```python
from build123d import *

# Parameters (mm, degrees)
ESQUISSE1_R        = 1.1
ESQUISSE1_W        = 6.844485425
ESQUISSE1_H        = 3
BOSS_EXTRU_1_DEPTH = 0.4
ESQUISSE3_W        = 10.5
ESQUISSE3_H        = 4.6
BOSS_EXTRU_3_DEPTH = 5.8
ESQUISSE4_W        = 3.029083023
ESQUISSE4_H        = 3
BOSS_EXTRU_4_DEPTH = 5
CONG_1_R           = 0.25


with BuildPart() as part:
    # Esquisse1 → Boss.-Extru.1 (new body)
    with BuildSketch(Plane.XY):
        with BuildLine():
            Line((-5.25, -2.9), (5.25, -2.9))
            Line((5.25, -2.9), (5.25, -2.4))
            Line((5.25, -2.4), (9.35, -2.4))
            ThreePointArc((9.35, -2.4), (9.703553391, -2.253553391), (9.85, -1.9))
            Line((9.85, -1.9), (9.85, 1.9))
            ThreePointArc((9.85, 1.9), (9.703553391, 2.253553391), (9.35, 2.4))
            Line((9.35, 2.4), (5.25, 2.4))
            Line((5.25, 2.4), (5.25, 2.9))
            Line((5.25, 2.9), (-5.25, 2.9))
            Line((-5.25, 2.9), (-5.25, 2.4))
            Line((-5.25, 2.4), (-9.35, 2.4))
            ThreePointArc((-9.35, 2.4), (-9.703553391, 2.253553391), (-9.85, 1.9))
            Line((-9.85, 1.9), (-9.85, -1.9))
            ThreePointArc((-9.85, -1.9), (-9.703553391, -2.253553391), (-9.35, -2.4))
            Line((-9.35, -2.4), (-5.25, -2.4))
            Line((-5.25, -2.4), (-5.25, -2.9))
        make_face()
        with Locations((-7.001967481, 0)):
            Circle(ESQUISSE1_R, mode=Mode.SUBTRACT)
        with Locations((6.936303644, 0)):
            Circle(ESQUISSE1_R, mode=Mode.SUBTRACT)
        with Locations((-0.061879176, 0)):
            Rectangle(ESQUISSE1_W, ESQUISSE1_H, mode=Mode.SUBTRACT)
    extrude(amount=BOSS_EXTRU_1_DEPTH)

    # Esquisse3 → Boss.-Extru.3 (add)
    with BuildSketch(Plane(origin=(0, 2.9, 0), x_dir=(1, 0, 0), z_dir=(0, 1, 0))):
        with Locations((0, -2.7)):
            Rectangle(ESQUISSE3_W, ESQUISSE3_H)
    extrude(amount=-BOSS_EXTRU_3_DEPTH)

    # Esquisse4 → Boss.-Extru.4 (add)
    with BuildSketch(Plane(origin=(0, 0, 0.4), x_dir=(-1, 0, 0), z_dir=(0, 0, -1))):
        with Locations((1.514541512, 0)):
            Rectangle(ESQUISSE4_W, ESQUISSE4_H)
    extrude(amount=BOSS_EXTRU_4_DEPTH)

    # Congé1
    cong_1_edges = [part.edges().sort_by_distance(p)[0] for p in [
        (-3.029083023, 0, -4.6),
        (0, 0, -4.6),
    ]]
    fillet(cong_1_edges, radius=CONG_1_R)


solid = part.part
```
Geometry: final body of the model. Coordinates: model frame, mm. A direction names the side the tool comes from. Round coordinates to 2 decimals unless told otherwise and drop trailing zeros. Write each loop counter-clockwise with the first axis right and the second up, starting at its lowest first coordinate (ties: lowest second). Pieces come first, ordered by that corner, then holes. Notation, with made-up numbers: M -16.5,50 L 7.5,50 A7 ccw 7.5,63 Z; hole C 80.5,51.5 d2. An arc over 180 degrees is marked long. Answer in a Markdown table with one row per item. Add a question column.
(1) Contact query for flat-ended pins moving along their axis: pin 1 (1.4 mm diameter, centred on x = -7.5, y = 0.5, fed in from +Z); pin 2 (2.5 mm diameter, centred on x = -1, z = -2, fed in from +Y); pin 3 (3.5 mm diameter, centred on x = -1, z = -2.5, fed in from -Y); pin 4 (1.8 mm diameter, centred on x = -7, y = 0, fed in from -Z). Output: stop coordinate, or through.
(2) Cut plane D-D, the plane z = 3.75. Return the cut outline in (x, y).
(3) Cut plane C-C, the plane y = -0.9. Return the cut outline in (x, z).
(4) Cut plane A-A, the plane y = 0. Return the cut outline in (x, z), then the cut area to 3 significant figures.
(5) Ray query, L1, parallel to Z at x = -3.25, y = -1; L2, parallel to Z at x = 6, y = -1.9; L3, parallel to X at y = -1.1, z = 1.5. Return the intervals inside material, ascending.
(6) Draft query along Y for faces 6 (the face through (-1, -1.5, -2)), 7 (the face through (-8.1, 0, 0.2)), 8 (the face through (7.986, 0.33, 0.197)), 9 (the face through (8, 1, 0.4)). Return one class per face: pulls with the +Y half, pulls with the -Y half, needs draft (parallel to the pull), parting line crosses it, or undercut.
(7) Cut plane B-B, the plane x = -1.5. Return the cut outline in (y, z), then the cut area to 3 significant figures.
(8) Reachability of faces 1 (the face through (0, 0, 5)), 2 (the face through (2, 0, 0.4)), 3 (the face through (-1, 1.5, -2)), 4 (the face through (-8, 1, 0.4)), 5 (the face through (0, -2.9, 2)) from +Z, -Z, +X, -X, +Y, -Y: full face, straight path, thin tool, end or side. Return the list, or none.
Established:
| question | item | result |
|---|---|---|
| 1 | pin 1 | z = 0.4 |
| 1 | pin 2 | y = 1.5 |
| 1 | pin 3 | y = -1.5 |
| 1 | pin 4 | through |
| 2 | outline | M -5.25,-2.9 L 5.25,-2.9 L 5.25,2.9 L -5.25,2.9 Z |
| 3 | outline | M -9.85,0 L -7.63,0 L -7.63,0.4 L -9.85,0.4 Z; M -6.37,0 L -3.48,0 L -3.48,0.4 L -3.03,0.4 L -3.03,-4.35 A0.25 ccw -2.78,-4.6 L -0.25,-4.6 A0.25 ccw 0,-4.35 L 0,0.4 L 3.36,0.4 L 3.36,0 L 6.3,0 L 6.3,0.4 L 5.25,0.4 L 5.25,5 L -5.25,5 L -5.25,0.4 L -6.37,0.4 Z; M 7.57,0 L 9.85,0 L 9.85,0.4 L 7.57,0.4 Z |
| 4 | outline | M -9.85,0 L -8.1,0 L -8.1,0.4 L -9.85,0.4 Z; M -5.9,0 L -3.48,0 L -3.48,0.4 L -3.03,0.4 L -3.03,-4.35 A0.25 ccw -2.78,-4.6 L -0.25,-4.6 A0.25 ccw 0,-4.35 L 0,0.4 L 3.36,0.4 L 3.36,0 L 5.84,0 L 5.84,0.4 L 5.25,0.4 L 5.25,5 L -5.25,5 L -5.25,0.4 L -5.9,0.4 Z; M 8.04,0 L 9.85,0 L 9.85,0.4 L 8.04,0.4 Z |
| 4 | area | 66.8 mm² |
| 5 | L1 | 0.4 to 5 |
| 5 | L2 | 0 to 0.4 |
| 5 | L3 | -5.25 to 5.25 |
| 6 | face 6 | pulls with the -Y half |
| 6 | face 7 | undercut |
| 6 | face 8 | undercut |
| 6 | face 9 | needs draft |
| 7 | outline | M -2.9,0 L -1.5,0 L -1.5,-4.6 L 1.5,-4.6 L 1.5,0 L 2.9,0 L 2.9,5 L -2.9,5 Z |
| 7 | area | 42.8 mm² |
| 8 | face 1 | +Z, +X, -X, +Y, -Y |
| 8 | face 2 | -Z |
| 8 | face 3 | -Z, +X, -X, +Y |
| 8 | face 4 | +Z, -X, +Y, -Y |
| 8 | face 5 | +Z, -Z, +X, -X, -Y |
